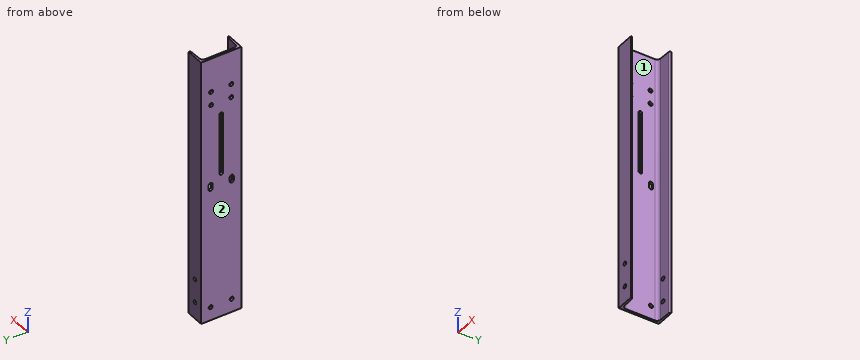
```python
from build123d import *

# Parameters (mm, degrees)
F1_DEPTH = 400
F2_R     = 6
F3_DEPTH = 55.001
F4_R     = 6
F5_DEPTH = 120.001


# Not quite as in the source:
# - a feature names something its author has since deleted; it is built from what else it names


with BuildPart() as f1:
    # F0 (on Top) → F1 (new body, symmetric)
    with BuildSketch(Plane.XY):
        with BuildLine():
            Line((0, 120), (0, 0))
            Line((0, 0), (55, 0))
            Line((55, 0), (55, 0.683595444))
            ThreePointArc((55, 0.683595444), (53.7475389551, 3.7986380977), (50.6873374512, 5.1796942729))
            Line((50.6873374512, 5.1796942729), (16.5836945529, 6.6006793936))
            ThreePointArc((16.5836945529, 6.6006793936), (9.7832467663, 9.6696931162), (7, 16.5920101246))
            Line((7, 16.5920101246), (7, 103.4079898754))
            ThreePointArc((7, 103.4079898754), (9.7832467663, 110.3303068838), (16.5836945529, 113.3993206064))
            Line((16.5836945529, 113.3993206064), (50.6873374512, 114.8203057271))
            ThreePointArc((50.6873374512, 114.8203057271), (53.7475389551, 116.2013619023), (55, 119.316404556))
            Line((55, 119.316404556), (55, 120))
            Line((55, 120), (0, 120))
        make_face()
    extrude(amount=F1_DEPTH, both=True)

    # F2 (on face) → F3 (cut, through all)
    with BuildSketch(Plane(origin=(0, 0, 0), x_dir=(0, -1, 0), z_dir=(-1, 0, 0))):
        with Locations((-90, 298)):
            Circle(F2_R)
        with Locations((-30, 298)):
            Circle(F2_R)
        with Locations((-30, 258)):
            Circle(F2_R)
        with Locations((-90, 258)):
            Circle(F2_R)
        with BuildLine():
            Line((-97.4973066239, 7.8202411081), (-97.4971376848, 8.1853094437))
            ThreePointArc((-97.4971376848, 8.1853094437), (-97.4999993576, 8.0027765611), (-97.4973066239, 7.8202411081))
        make_face()
        with Locations((-91.5, -360)):
            Circle(F2_R)
        with Locations((-28.5, -360)):
            Circle(F2_R)
        with BuildLine():
            Line((-97.4945650308, 13.7446764959), (-97.4971376848, 8.1853094437))
            Line((-97.4971376848, 8.1853094437), (-97.4973066239, 7.8202411081))
            Line((-97.4973066239, 7.8202411081), (-97.4999974302, 2.0055531216))
            ThreePointArc((-97.4999974302, 2.0055531216), (-97.4999993576, 2.0027765611), (-97.5, 2))
            ThreePointArc((-97.5, 2), (-91.5, -4), (-85.5, 2))
            Line((-85.5, 2), (-85.5, 14))
            ThreePointArc((-85.5, 14), (-91.6276906718, 19.9986411038), (-97.4945650308, 13.7446764959))
        make_face()
        with BuildLine():
            Line((-22.5, 2), (-22.5, 14))
            ThreePointArc((-22.5, 14), (-28.5, 20), (-34.5, 14))
            Line((-34.5, 14), (-34.5, 2))
            ThreePointArc((-34.5, 2), (-28.5, -4), (-22.5, 2))
        make_face()
        with BuildLine():
            Line((-65.5, 218), (-65.5, 38))
            ThreePointArc((-65.5, 38), (-60, 32.5), (-54.5, 38))
            Line((-54.5, 38), (-54.5, 218))
            ThreePointArc((-54.5, 218), (-60, 223.5), (-65.5, 218))
        make_face()
    extrude(amount=-F3_DEPTH, mode=Mode.SUBTRACT)

    # F4 (on face) → F5 (cut, through all)
    with BuildSketch(Plane.XZ):
        with Locations((27.5, -280)):
            Circle(F4_R)
        with Locations((27.5, -350)):
            Circle(F4_R)
    extrude(amount=-F5_DEPTH, mode=Mode.SUBTRACT)


solid = f1.part
```
Input: part model. Units: mm. Frame: model coordinates. Face numbers are marked on the shaded views. A direction names the side the tool comes from. Coordinates: 2 decimals unless noted, no trailing zeros. Loops run counter-clockwise (first coordinate to the right, second up) from the corner with the lowest first, then second, coordinate; pieces in that order, holes last. Notation, with made-up numbers: (14, 27) - (43, 27) arc R17 ccw to (43, 49) - close; hole circle Ø2 at (-15, 29). An arc over 180 degrees is marked (long way). Answer in a Markdown table with one row per item.
(1) Cut plane B-B on z = -47.5. Output: boundary loops of the cut face in (x, y), plus the area to 3 significant figures.
Model answer:
| item | result |
|---|---|
| outline | (0, 0) - (55, 0) - (55, 0.68) arc R4.5 ccw to (50.69, 5.18) - (16.58, 6.6) arc R10 cw to (7, 16.59) - (7, 103.41) arc R10 cw to (16.58, 113.4) - (50.69, 114.82) arc R4.5 ccw to (55, 119.32) - (55, 120) - (0, 120) - close |
| area | 1,450 mm² |
(2) Set-up query: the marked faces 1 and 2. Return all of +Z, -Z, +X, -X, +Y, -Y with unobstructed straight access to the full face (end or side cutting, diameter ignored); none if empty.
Model answer:
| item | result |
|---|---|
| face 1 | +Z, -Z, +X |
| face 2 | +Z, -Z, -X, +Y, -Y |
(3) Pin query (flat end, axial travel): P1, Ø14, axis at x = 27.5, z = -280, coming from the -Y side; P2, Ø19, axis at y = 91.5, z = -360, coming from the +X side. Return the tip coordinate at first contact, or that it passes through.
Model answer:
| item | result |
|---|---|
| P1 | stops at y = 0 |
| P2 | stops at x = 7 |
(4) Cut plane A-A on z = 200. Output: boundary loops of the cut face in (x, y), plus the area to 3 significant figures.
Model answer:
| item | result |
|---|---|
| outline | (0, 0) - (55, 0) - (55, 0.68) arc R4.5 ccw to (50.69, 5.18) - (16.58, 6.6) arc R10 cw to (7, 16.59) - (7, 54.5) - (0, 54.5) - close; (0, 65.5) - (7, 65.5) - (7, 103.41) arc R10 cw to (16.58, 113.4) - (50.69, 114.82) arc R4.5 ccw to (55, 119.32) - (55, 120) - (0, 120) - close |
| area | 1,370 mm² |
(5) Material intervals for L1, parallel to Y at x = 3, z = 258; L2, parallel to Y at x = 16.5, z = -106; L3, parallel to Z at x = 2.5, y = 30, sorted ascending. Write a range as from..to.
Model answer:
| item | result |
|---|---|
| L1 | y = 0..24, 36..84, 96..120 |
| L2 | y = 0..6.6, 113.4..120 |
| L3 | z = -400..-365.81, -354.19..-3.81, 19.81..252, 264..292, 304..400 |
